Can you work these out from the model? Positions are in its coordinate system, mm. A direction names the side the tool comes from. Coordinates: 2 decimals unless noted, no trailing zeros. Order: outer loops, then holes, each group sorted by start corner. A loop starts at its lowest first (then second) coordinate and runs counter-clockwise, first axis right, second up.
```python
from build123d import *

# Parameters (mm, degrees)
SKETCH_1_W          = 70
SKETCH_1_H          = 70
SKETCH_1_R          = 1.6
EXTRUDE_1_DEPTH     = 1
EXTRUDE_2_DEPTH     = 1
SKETCH_5_R          = 1.55
CUT_EXTRUDE_1_DEPTH = 10
SKETCH_6_R          = 1.55
CUT_EXTRUDE_2_DEPTH = 10
CHAMFER_1_SIZE      = 10
FILLET_1_R          = 2


with BuildPart() as part:
    # 草图1 → 凸台-拉伸1 (new body)
    with BuildSketch(Plane(origin=(0, 0, 0), x_dir=(1, 0, 0), z_dir=(0, 1, 0))):
        Rectangle(SKETCH_1_W, SKETCH_1_H)
        with Locations(Location((13, -13, 0), (0, 0, 270))):
            Circle(SKETCH_1_R, mode=Mode.SUBTRACT)
        with Locations(Location((13, 13, 0), (0, 0, 270))):
            Circle(SKETCH_1_R, mode=Mode.SUBTRACT)
        with Locations(Location((-13, 13, 0), (0, 0, 270))):
            Circle(SKETCH_1_R, mode=Mode.SUBTRACT)
        with Locations(Location((-13, -13, 0), (0, 0, 270))):
            Circle(SKETCH_1_R, mode=Mode.SUBTRACT)
    extrude(amount=EXTRUDE_1_DEPTH)

    # 草图2 → 凸台-拉伸2 (add)
    with BuildSketch(Plane.XZ):
        Polygon((35, -35), (35, -69), (20, -84), (-90, -84), (-100, -74), (-189, -74), (-189, -36.5), (-57, -36.5), (-57, 36.5), (-218, 36.5), (-218, 74), (-100, 74), (-90, 84), (20, 84), (35, 69), (35, 35), (-35, 35), (-35, -35), align=None)
    extrude(amount=-EXTRUDE_2_DEPTH)

    # 草图5 → 切除-拉伸1 (cut)
    with BuildSketch(Plane(origin=(0, 1, 0), x_dir=(1, 0, 0), z_dir=(0, 1, 0))):
        with Locations(Location((-146.3, -39.25, 0), (0, 0, 270))):
            Circle(SKETCH_5_R)
        with Locations(Location((-136.3, 39.25, 0), (0, 0, 270))):
            Circle(SKETCH_5_R)
    extrude(amount=-CUT_EXTRUDE_1_DEPTH, mode=Mode.SUBTRACT)

    # 草图6 → 切除-拉伸2 (cut)
    with BuildSketch(Plane.XZ):
        with Locations(Location((28.9, 51.8, 0), (0, 0, 270))):
            Circle(SKETCH_6_R)
        with Locations(Location((28.9, 38.2, 0), (0, 0, 270))):
            Circle(SKETCH_6_R)
        with Locations(Location((28.9, -51.8, 0), (0, 0, 270))):
            Circle(SKETCH_6_R)
        with Locations(Location((28.9, -38.2, 0), (0, 0, 270))):
            Circle(SKETCH_6_R)
        with Locations(Location((-5, 80, 0), (0, 0, 270))):
            Circle(SKETCH_6_R)
        with Locations(Location((-25, 80, 0), (0, 0, 270))):
            Circle(SKETCH_6_R)
        with Locations(Location((-132, 70, 0), (0, 0, 270))):
            Circle(SKETCH_6_R)
        with Locations(Location((-152, 70, 0), (0, 0, 270))):
            Circle(SKETCH_6_R)
        with Locations(Location((-144, -70, 0), (0, 0, 270))):
            Circle(SKETCH_6_R)
        with Locations(Location((-164, -70, 0), (0, 0, 270))):
            Circle(SKETCH_6_R)
        with Locations(Location((-5, -80, 0), (0, 0, 270))):
            Circle(SKETCH_6_R)
        with Locations(Location((-25, -80, 0), (0, 0, 270))):
            Circle(SKETCH_6_R)
        with Locations(Location((-45, 80, 0), (0, 0, 270))):
            Circle(SKETCH_6_R)
        with Locations(Location((-65, 80, 0), (0, 0, 270))):
            Circle(SKETCH_6_R)
        with Locations(Location((-45, -80, 0), (0, 0, 270))):
            Circle(SKETCH_6_R)
        with Locations(Location((-65, -80, 0), (0, 0, 270))):
            Circle(SKETCH_6_R)
        with Locations(Location((-192, 70, 0), (0, 0, 270))):
            Circle(SKETCH_6_R)
        with Locations(Location((-172, 70, 0), (0, 0, 270))):
            Circle(SKETCH_6_R)
    extrude(amount=-CUT_EXTRUDE_2_DEPTH, mode=Mode.SUBTRACT)

    # 倒角1
    chamfer_1_edges = [part.edges().sort_by_distance(p)[0] for p in [
        (-57, 0.5, -36.5),
        (-57, 0.5, 36.5),
    ]]
    chamfer(chamfer_1_edges, length=CHAMFER_1_SIZE)

    # 圆角1
    fillet_1_edges = [part.edges().sort_by_distance(p)[0] for p in [
        (-57, 0.5, 26.5),
        (-57, 0.5, -26.5),
        (-67, 0.5, -36.5),
        (-67, 0.5, 36.5),
        (35, 0.5, -69),
        (20, 0.5, -84),
        (-90, 0.5, -84),
        (-100, 0.5, -74),
        (-189, 0.5, -74),
        (-189, 0.5, -36.5),
        (-218, 0.5, 36.5),
        (-218, 0.5, 74),
        (-100, 0.5, 74),
        (-90, 0.5, 84),
        (20, 0.5, 84),
        (35, 0.5, 69),
    ]]
    fillet(fillet_1_edges, radius=FILLET_1_R)


solid = part.part
```
1. Thinking about a two-plate mould opening in Z: for faces 3 (the flat face through (-34, 1, 1)), 4 (the flat face through (-61.9, 0.5, -31.4)), 5 (the flat face through (-95.1, 0.5, 78.9)), which applies, pulls with the +Z half, pulls with the -Z half, needs draft (parallel to the pull), parting line crosses it, or undercut?
Completed:
face 3: needs draft
face 4: undercut
face 5: pulls with the +Z half
2. I'm going to push a flat-ended pin straight in: pin 1 (0.5 mm diameter, centred on y = 0.5, z = -52, fed in from -X). Where does the tip first touch, or does it pass through?
Completed:
pin 1: stops at x = -189
3. On a 3-axis mill with a long thin cutter (end or side, diameter ignored), from which of +Z, -Z, +X, -X, +Y, -Y can I reach the whole of each face in a straight line? I mean faces 1 (the flat face through (-94.9, 0.5, -79.1)), 2 (the flat face through (-62.1, 0.5, 31.6)). Say none if no direction works.
Completed:
face 1: -Z, -X, +Y, -Y
face 2: -X, +Y, -Y
4. Imagine slicing it at B-B on z = -58.5. Please give me the cut outline in (x, y), then the cut area to 3 significant figures.
Completed:
outline: (-189, 0) - (35, 0) - (35, 1) - (-189, 1) - close
area: 224 mm2
5. Please list where these lines run through material, in increasing order: probe 1 along Z at (x, y) = (-144, 0.5); probe 2 along Z at (x, y) = (-163, 0.4); probe 3 along Z at (x, y) = (-174, 0.15).
Completed:
probe 1: z = -74 to -71.55, -68.45 to -36.5, 36.5 to 74
probe 2: z = -74 to -71.18, -68.82 to -36.5, 36.5 to 74
probe 3: z = -74 to -36.5, 36.5 to 74
6. Imagine slicing it at A-A on y = 0.8. Give the number of separate pieces and of enclosed holes in the cut face, then the cut area to 3 significant figures.
Completed:
separate pieces: 1
enclosed holes: 24
area: 26,900 mm2
